Could you check a few things on this model? Use its own coordinates, in mm. Coordinates: 2 decimals unless noted, no trailing zeros. Write each loop counter-clockwise with the first axis right and the second up, starting at its lowest first coordinate (ties: lowest second). Pieces come first, ordered by that corner, then holes. Notation, with made-up numbers: M 24,-24.5 L 57,-24.5 A17 ccw 57,-20.5 Z; hole C -7.5,31.5 d11. An arc over 180 degrees is marked long. Answer as CSV lines item,"result". Start each with the question number.
Item 1: If I drill on line 1 along Z through (x, y) = (-2.5, 1.5); line 2 along Y through (x, z) = (-6.75, 22.5); line 3 along Y through (x, z) = (-7, 19), over which ranges is the centre line in solid material (lowest first)? Write a range as [from, to].
Item 2: Suppose I cut it at C-C, the plane y = -16. Write out the boundary of the cut face in (x, z).
Item 3: Suppose I cut it at A-A, the plane x = 0. Write out the boundary of the cut face in (y, z).
Item 4: Suppose I cut it at B-B, the plane z = 23. Write out the boundary of the cut face in (x, y) (1 decimal), and give its area (3 significant figures).
Item 5: Suppose I cut it at D-D, the plane y = -21.5. Write out the boundary of the cut face in (x, z), and give its area (3 significant figures).
Item 6: I'm going to push flat-ended pins straight in: P1, Ø12, axis at x = 7.5, z = 13.5, coming from the +Y side; P2, Ø6, axis at x = 9.5, z = 21.5, coming from the +Y side; P3, Ø4, axis at y = -18, z = 4, coming from the +X side. Where does each tip first touch, or does it pass through?
```python
from build123d import *

# Parameters (mm, degrees)
F1_DEPTH = 32
F0_R     = 4
F0_R_2   = 4.8981963292
F0_R_3   = 2.949247213
F0_R_4   = 2.5
F0_R_5   = 1.5
F0_W     = 2.8284271247
F0_H     = 2.8284271247
F0_W_2   = 1.767766953
F0_H_2   = 1.767766953
F2_DEPTH = 2
F3_DEPTH = 3
F4_DEPTH = 6


with BuildPart() as f1:
    # F0 (on Top) → F1 (new body)
    with BuildSketch(Plane.XY):
        with BuildLine():
            Line((9.9107124982, -31.3333333333), (13.8749974975, -1.8666666667))
            ThreePointArc((13.8749974975, -1.8666666667), (7.2404165941, 11.9823356464), (-8.1052915892, 11.4150886223))
            Line((-8.1052915892, 11.4150886223), (-6.9473927907, 9.7843616762))
            ThreePointArc((-6.9473927907, 9.7843616762), (5.5059643348, 10.6622866565), (12, 0))
            ThreePointArc((12, 0), (11.9731837866, -0.8017917516), (11.8928549979, -1.6))
            Line((11.8928549979, -1.6), (9.843423449, -16.8334951494))
            Line((9.843423449, -16.8334951494), (9.6796856306, -18.0505639815))
            Line((9.6796856306, -18.0505639815), (9.0834008366, -22.4827693518))
            Line((9.0834008366, -22.4827693518), (8.9196630183, -23.6998381839))
            Line((8.9196630183, -23.6998381839), (7.9285699986, -31.0666666667))
            ThreePointArc((7.9285699986, -31.0666666667), (0, -38), (-7.9285699986, -31.0666666667))
            Line((-7.9285699986, -31.0666666667), (-8.9196630183, -23.6998381839))
            Line((-8.9196630183, -23.6998381839), (-9.0834008366, -22.4827693518))
            Line((-9.0834008366, -22.4827693518), (-9.6796856306, -18.0505639815))
            Line((-9.6796856306, -18.0505639815), (-9.843423449, -16.8334951494))
            Line((-9.843423449, -16.8334951494), (-11.892854985, -1.6000000955))
            ThreePointArc((-11.892854985, -1.6000000955), (-11.9601461079, 0.9771924467), (-11.4754059318, 3.5092817927))
            Line((-11.4754059318, 3.5092817927), (-13.3879735871, 4.0941620915))
            ThreePointArc((-13.3879735871, 4.0941620915), (-13.953503788, 1.1400579105), (-13.8749974975, -1.8666666667))
            Line((-13.8749974975, -1.8666666667), (-9.9107124982, -31.3333333333))
            ThreePointArc((-9.9107124982, -31.3333333333), (0, -40), (9.9107124982, -31.3333333333))
        make_face()
    extrude(amount=F1_DEPTH)

    # F0 (on Top) → F2 (join)
    with BuildSketch(Plane.XY):
        with BuildLine():
            ThreePointArc((12, 0), (5.5059643348, 10.6622866565), (-6.9473927907, 9.7843616762))
            ThreePointArc((-6.9473927907, 9.7843616762), (-9.7310860174, 7.0218206272), (-11.4754059318, 3.5092817927))
            ThreePointArc((-11.4754059318, 3.5092817927), (-11.9601461079, 0.9771924467), (-11.892854985, -1.6000000955))
            ThreePointArc((-11.892854985, -1.6000000955), (4.82e-08, -12), (11.8928549979, -1.6))
            ThreePointArc((11.8928549979, -1.6), (11.9731837866, -0.8017917516), (12, 0))
        make_face()
        Circle(F0_R, mode=Mode.SUBTRACT)
        with BuildLine():
            ThreePointArc((8, -30), (-0.5345278344, -22.0178774756), (-7.9285699986, -31.0666666667))
            ThreePointArc((-7.9285699986, -31.0666666667), (0, -38), (7.9285699986, -31.0666666667))
            ThreePointArc((7.9285699986, -31.0666666667), (7.9821225244, -30.5345278344), (8, -30))
        make_face()
        with Locations((0, -30)):
            Circle(F0_R_2, mode=Mode.SUBTRACT)
        with BuildLine():
            ThreePointArc((11.8928549979, -1.6), (4.82e-08, -12), (-11.892854985, -1.6000000955))
            Line((-11.892854985, -1.6000000955), (-9.843423449, -16.8334951494))
            ThreePointArc((-9.843423449, -16.8334951494), (-3.4351157347, -19.4666666667), (-8.9196630183, -23.6998381839))
            Line((-8.9196630183, -23.6998381839), (-7.9285699986, -31.0666666667))
            ThreePointArc((-7.9285699986, -31.0666666667), (-0.5345278344, -22.0178774756), (8, -30))
            ThreePointArc((8, -30), (7.9821225244, -30.5345278344), (7.9285699986, -31.0666666667))
            Line((7.9285699986, -31.0666666667), (8.9196630183, -23.6998381839))
            ThreePointArc((8.9196630183, -23.6998381839), (3.4351157347, -19.4666666667), (9.843423449, -16.8334951494))
            Line((9.843423449, -16.8334951494), (11.8928549979, -1.6))
        make_face()
        with Locations((0, -30)):
            Circle(F0_R_2)
        with Locations((0, -30)):
            Circle(F0_R_3, mode=Mode.SUBTRACT)
        Circle(F0_R)
        Circle(F0_R_4, mode=Mode.SUBTRACT)
        with Locations((0, -30)):
            Circle(F0_R_3)
        with Locations((0, -30)):
            Circle(F0_R_5, mode=Mode.SUBTRACT)
        with BuildLine():
            ThreePointArc((-9.0834008366, -22.4827693518), (-4.4261869845, -19.6), (-9.6796856306, -18.0505639815))
            Line((-9.6796856306, -18.0505639815), (-9.0834008366, -22.4827693518))
        make_face()
        with BuildLine():
            Line((9.0834008366, -22.4827693518), (9.6796856306, -18.0505639815))
            ThreePointArc((9.6796856306, -18.0505639815), (4.4261869845, -19.6), (9.0834008366, -22.4827693518))
        make_face()
        Circle(F0_R_4)
        Rectangle(F0_W, F0_H, mode=Mode.SUBTRACT)
        with BuildLine():
            Line((9.6796856306, -18.0505639815), (9.843423449, -16.8334951494))
            ThreePointArc((9.843423449, -16.8334951494), (3.4351157347, -19.4666666667), (8.9196630183, -23.6998381839))
            Line((8.9196630183, -23.6998381839), (9.0834008366, -22.4827693518))
            ThreePointArc((9.0834008366, -22.4827693518), (4.4261869845, -19.6), (9.6796856306, -18.0505639815))
        make_face()
        with BuildLine():
            ThreePointArc((-8.9196630183, -23.6998381839), (-3.4351157347, -19.4666666667), (-9.843423449, -16.8334951494))
            Line((-9.843423449, -16.8334951494), (-9.6796856306, -18.0505639815))
            ThreePointArc((-9.6796856306, -18.0505639815), (-4.4261869845, -19.6), (-9.0834008366, -22.4827693518))
            Line((-9.0834008366, -22.4827693518), (-8.9196630183, -23.6998381839))
        make_face()
        Rectangle(F0_W, F0_H)
        with Locations((0, -30)):
            Circle(F0_R_5)
        with Locations((0, -30)):
            Rectangle(F0_W_2, F0_H_2, mode=Mode.SUBTRACT)
        with Locations((0, -30)):
            Rectangle(F0_W_2, F0_H_2)
    extrude(amount=F2_DEPTH)

    # F0 (on Top) → F3 (cut)
    with BuildSketch(Plane.XY):
        Rectangle(F0_W, F0_H)
    extrude(amount=F3_DEPTH, mode=Mode.SUBTRACT)

    # F0 (on Top) → F4 (join)
    with BuildSketch(Plane.XY):
        with Locations((0, -30)):
            Circle(F0_R_5)
        with Locations((0, -30)):
            Rectangle(F0_W_2, F0_H_2, mode=Mode.SUBTRACT)
    extrude(amount=F4_DEPTH)


solid = f1.part
```
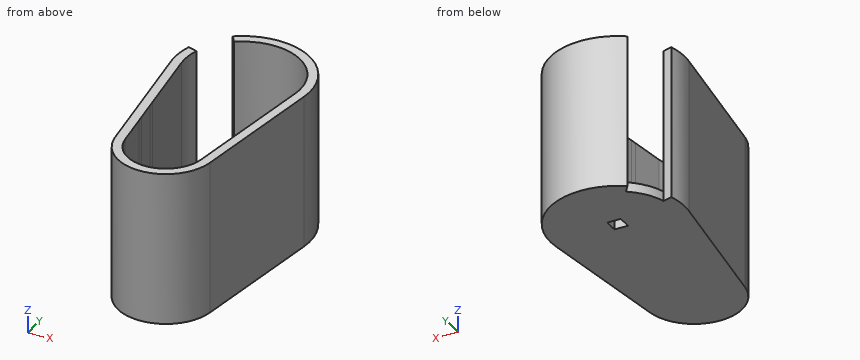
Ans:
1,line 1,"z = [0, 2]"
1,line 2,"y = [-37.38, -34.29], [9.92, 12.27]"
1,line 3,"y = [-37.14, -33.87], [9.86, 12.12]"
2,outline,"M -11.97,0 L 11.97,0 L 11.97,32 L 9.96,32 L 9.96,2 L -9.96,2 L -9.96,32 L -11.97,32 Z"
3,outline,"M -40,0 L -1.41,0 L -1.41,2 L -28.5,2 L -28.5,6 L -29.12,6 L -29.12,2 L -30.88,2 L -30.88,6 L -31.5,6 L -31.5,2 L -38,2 L -38,32 L -40,32 Z; M 1.41,0 L 14,0 L 14,32 L 12,32 L 12,2 L 1.41,2 Z"
4,outline,"M -13.9,-1.9 L -9.9,-31.3 A10 ccw 9.9,-31.3 L 13.9,-1.9 A14 ccw -8.1,11.4 L -6.9,9.8 A12 cw 11.9,-1.6 L 7.9,-31.1 A8 cw -7.9,-31.1 L -11.9,-1.6 A12 cw -11.5,3.5 L -13.4,4.1 A14 ccw Z"
4,area,"242 mm^2"
5,outline,"M -11.23,0 L 11.23,0 L 11.23,32 L 9.22,32 L 9.22,2 L -9.22,2 L -9.22,32 L -11.23,32 Z"
5,area,"166 mm^2"
6,P1,"stops at y = 13.92"
6,P2,"stops at y = 12.4"
6,P3,"stops at x = 11.97"
